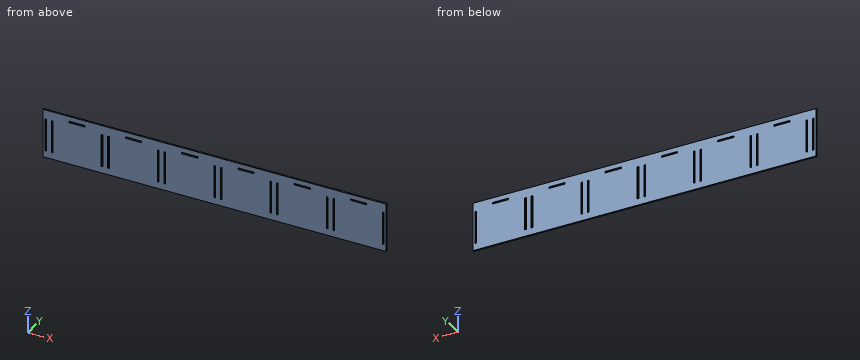
from build123d import *

# Parameters (mm, degrees)
SKETCH1_W           = 424
SKETCH1_H           = 60
SKETCH1_W_2         = 2
SKETCH1_H_2         = 40.5
SKETCH1_W_3         = 20
SKETCH1_H_3         = 2
BOSS_EXTRUDE2_DEPTH = 2


with BuildPart() as part:
    # Sketch1 → Boss-Extrude2 (new body)
    with BuildSketch(Plane(origin=(0, 0, 0), x_dir=(1, 0, 0), z_dir=(0, 1, 0))):
        with Locations((212, -30)):
            Rectangle(SKETCH1_W, SKETCH1_H)
        with Locations((80.95, -28.5)):
            Rectangle(SKETCH1_W_2, SKETCH1_H_2, mode=Mode.SUBTRACT)
        with Locations((150.5, -28.5)):
            Rectangle(SKETCH1_W_2, SKETCH1_H_2, mode=Mode.SUBTRACT)
        with Locations((3.35, -28.5)):
            Rectangle(SKETCH1_W_2, SKETCH1_H_2, mode=Mode.SUBTRACT)
        with Locations((72.9, -28.5)):
            Rectangle(SKETCH1_W_2, SKETCH1_H_2, mode=Mode.SUBTRACT)
        with Locations((11.4, -28.5)):
            Rectangle(SKETCH1_W_2, SKETCH1_H_2, mode=Mode.SUBTRACT)
        with Locations((359.15, -28.5)):
            Rectangle(SKETCH1_W_2, SKETCH1_H_2, mode=Mode.SUBTRACT)
        with Locations((351.1, -28.5)):
            Rectangle(SKETCH1_W_2, SKETCH1_H_2, mode=Mode.SUBTRACT)
        with Locations((289.6, -28.5)):
            Rectangle(SKETCH1_W_2, SKETCH1_H_2, mode=Mode.SUBTRACT)
        with Locations((220.05, -28.5)):
            Rectangle(SKETCH1_W_2, SKETCH1_H_2, mode=Mode.SUBTRACT)
        with Locations((142.45, -28.5)):
            Rectangle(SKETCH1_W_2, SKETCH1_H_2, mode=Mode.SUBTRACT)
        with Locations((111.7, -53.2)):
            Rectangle(SKETCH1_W_3, SKETCH1_H_3, mode=Mode.SUBTRACT)
        with Locations((42.15, -53.2)):
            Rectangle(SKETCH1_W_3, SKETCH1_H_3, mode=Mode.SUBTRACT)
        with Locations((212, -28.5)):
            Rectangle(SKETCH1_W_2, SKETCH1_H_2, mode=Mode.SUBTRACT)
        with Locations((281.55, -28.5)):
            Rectangle(SKETCH1_W_2, SKETCH1_H_2, mode=Mode.SUBTRACT)
        with Locations((181.25, -53.2)):
            Rectangle(SKETCH1_W_3, SKETCH1_H_3, mode=Mode.SUBTRACT)
        with Locations((250.8, -53.2)):
            Rectangle(SKETCH1_W_3, SKETCH1_H_3, mode=Mode.SUBTRACT)
        with Locations((420.65, -28.5)):
            Rectangle(SKETCH1_W_2, SKETCH1_H_2, mode=Mode.SUBTRACT)
        with Locations((320.35, -53.2)):
            Rectangle(SKETCH1_W_3, SKETCH1_H_3, mode=Mode.SUBTRACT)
        with Locations((389.9, -53.2)):
            Rectangle(SKETCH1_W_3, SKETCH1_H_3, mode=Mode.SUBTRACT)
    extrude(amount=BOSS_EXTRUDE2_DEPTH)


solid = part.part
Geometry: final body of the model. Coordinates: model frame, mm. Round coordinates to 2 decimals unless told otherwise and drop trailing zeros. Order: outer loops, then holes, each group sorted by start corner. A loop starts at its lowest first (then second) coordinate and runs counter-clockwise, first axis right, second up. Notation, with made-up numbers: (63, 45.25) - (87, 45.25) arc R13 cw to (87, 54.25) - close; hole circle Ø6 at (46, 79.5). An arc over 180 degrees is marked (long way). Write each question's results on one line, items separated by ' | '.
Item 1: Section B-B, the plane z = 26. State how many separate pieces and enclosed holes the cut face has, and give its area (3 significant figures).
Completed:
separate pieces: 14 | enclosed holes: 0 | area: 796 mm^2
Item 2: Material intervals for line 1 along Z through (x, y) = (251, 1); line 2 along Z through (x, y) = (290, 0.9), sorted ascending. Write a range as [from, to].
Completed:
line 1: [0, 52.2], [54.2, 60] | line 2: [0, 8.25], [48.75, 60]
Item 3: Section A-A, the plane x = 250. Return the cut outline in (y, z).
Completed:
outline: (0, 0) - (2, 0) - (2, 52.2) - (0, 52.2) - close; (0, 54.2) - (2, 54.2) - (2, 60) - (0, 60) - close
Item 4: First-contact query: pin 1 Ø4 at (x, z) = (348, 36) entering from -Y. Flat tip, straight axial feed; report the tip coordinate or a pass-through.
Completed:
pin 1: y = 0
